For this review, use the dimensioned drawing (mm, ordinates from the lowest corner) and the shaded views. A direction names the side the tool comes from. Give positions to 0.01 mm unless a question says otherwise; leave off trailing zeros. Loops run counter-clockwise (first coordinate to the right, second up) from the corner with the lowest first, then second, coordinate; pieces in that order, holes last. Notation, with made-up numbers: (3.5, -1.75) -> (38.5, -1.75) arc R9 cw to (38.5, 15.25) -> close; hole circle Ø6 at (75.25, -37). An arc over 180 degrees is marked (long way). Use a Markdown table: item, result. Add a question column.
1. Add section B-B (y = 50.5). State the section outline as (x, z) points, and give its area (3 significant figures).
2. Add section D-D (x = 17.5). State the section outline as (y, z) points, and give its area (3 significant figures).
3. Draft analysis for pull direction X (two halves, no side actions). For the marked faces 4, 5 and 6, state which applies: pulls with the +X half, pulls with the -X half, needs draft (parallel to the pull), parting line crosses it, or undercut.
4. For the marked faces 1, 2 and 3, list the 3-axis set-ups (+Z, -Z, +X, -X, +Y, -Y) from which the entire face can be reached by the end or side of a thin tool; tool diameter is ignored.
5. To check wall thickness, follow line 1 (X direction, y = 70, z = 6); line 2 (X direction, y = 53, z = 1.5); line 3 (Z direction, x = 35, y = 123). State the ranges of each line that lie inside material, in increasing order.
6. Add section C-C (x = 50). State the section outline as (y, z) points.
7. Add section A-A (z = 7). State the section outline as (x, y) points, and give its area (3 significant figures).
8. For pin 1 Ø3 at (y, z) = (92, 7.5) entering from +X; pin 2 Ø3 at (y, z) = (107.5, 2.5) entering from +X; pin 3 Ø3 at (y, z) = (109, 8.5) entering from -X, all flat-tipped, find the tip position at first contact; note any pin that passes through.
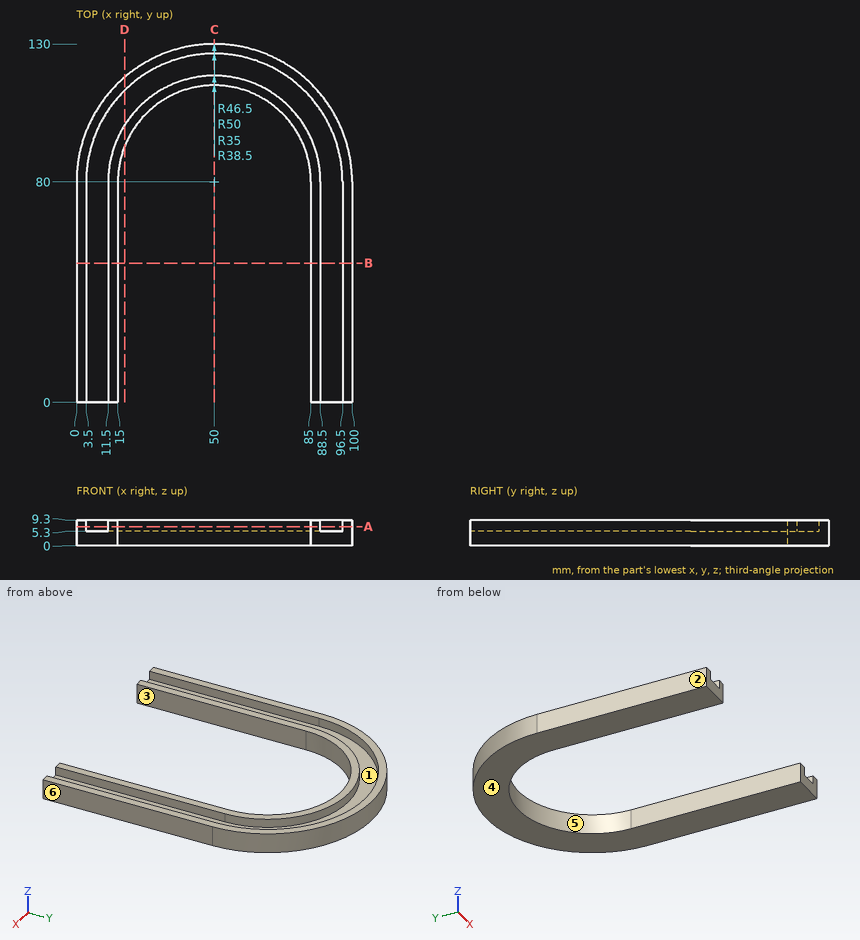
Taken from the geometry:
| question | item | result |
|---|---|---|
| 1 | outline | (0, 0) -> (15, 0) -> (15, 9.3) -> (11.5, 9.3) -> (11.5, 5.3) -> (3.5, 5.3) -> (3.5, 9.3) -> (0, 9.3) -> close; (85, 0) -> (100, 0) -> (100, 9.3) -> (96.5, 9.3) -> (96.5, 5.3) -> (88.5, 5.3) -> (88.5, 9.3) -> (85, 9.3) -> close |
| 1 | area | 215 mm^2 |
| 2 | outline | (92.99, 0) -> (118, 0) -> (118, 9.3) -> (113.26, 9.3) -> (113.26, 5.3) -> (100.64, 5.3) -> (100.64, 9.3) -> (92.99, 9.3) -> close |
| 2 | area | 182 mm^2 |
| 3 | face 4 | needs draft |
| 3 | face 5 | undercut |
| 3 | face 6 | pulls with the +X half |
| 4 | face 1 | +Z |
| 4 | face 2 | +Z, -Z, -X, +Y, -Y |
| 4 | face 3 | +Z, -Z, -Y |
| 5 | line 1 | x = 0 to 3.5, 11.5 to 15, 85 to 88.5, 96.5 to 100 |
| 5 | line 2 | x = 0 to 15, 85 to 100 |
| 5 | line 3 | z = 0 to 5.3 |
| 6 | outline | (115, 0) -> (130, 0) -> (130, 9.3) -> (126.5, 9.3) -> (126.5, 5.3) -> (118.5, 5.3) -> (118.5, 9.3) -> (115, 9.3) -> close |
| 7 | outline | (0, 0) -> (3.5, 0) -> (3.5, 80) arc R46.5 cw to (96.5, 80) -> (96.5, 0) -> (100, 0) -> (100, 80) arc R50 ccw to (0, 80) -> close; (11.5, 0) -> (15, 0) -> (15, 80) arc R35 cw to (85, 80) -> (85, 0) -> (88.5, 0) -> (88.5, 80) arc R38.5 ccw to (11.5, 80) -> close |
| 7 | area | 2,050 mm^2 |
| 8 | pin 1 | stops at x = 98.89 |
| 8 | pin 2 | stops at x = 92.71 |
| 8 | pin 3 | stops at x = 8.24 |
